Can you work these out from the drawing? Everything is in mm from the part's minimum corner. Round coordinates to 2 decimals unless told otherwise and drop trailing zeros. Loops run counter-clockwise (first coordinate to the right, second up) from the corner with the lowest first, then second, coordinate; pieces in that order, holes last. Notation, with made-up numbers: M 87.25,7 L 118.25,7 A31 cw 118.25,41 Z; hole C -27.5,62 d2. An arc over 180 degrees is marked long. Use a Markdown table: item, result.
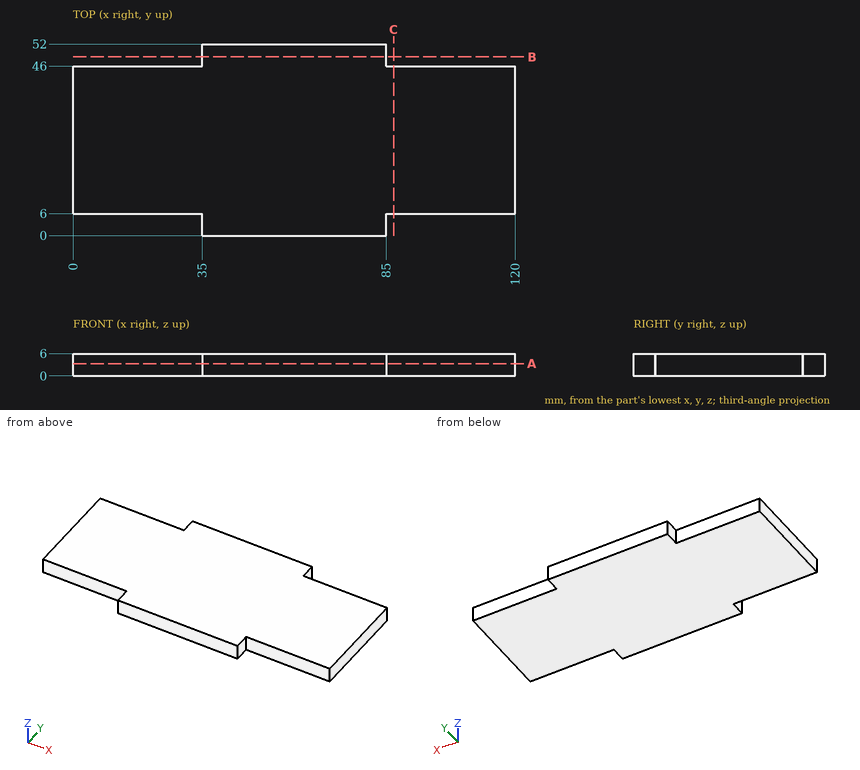
1. I need wall thicknesses on probe 1 along Y at (x, z) = (103, 4.15). Which ranges of the line are inside material? Lowest first, please. Write a range as from..to.
Answer sheet:
| item | result |
|---|---|
| probe 1 | 6..46 |
2. For pin 1 Ø3 at (x, z) = (9, 4.5) entering from -Y; pin 2 Ø3 at (y, z) = (48, 3) entering from -X; pin 3 Ø1 at (x, z) = (103.5, 2.5) entering from +Y, each with a flat end and sliding along its axis, tell me the tip position at first contact or that it passes through.
Answer sheet:
| item | result |
|---|---|
| pin 1 | y = 6 |
| pin 2 | x = 35 |
| pin 3 | y = 46 |
3. Imagine slicing it at B-B, the plane y = 48.5. Write out the boundary of the cut face in (x, z), then the cut area to 3 significant figures.
Answer sheet:
| item | result |
|---|---|
| outline | M 35,0 L 85,0 L 85,6 L 35,6 Z |
| area | 300 mm2 |
4. Imagine slicing it at C-C, the plane x = 87. Write out the boundary of the cut face in (y, z), then the cut area to 3 significant figures.
Answer sheet:
| item | result |
|---|---|
| outline | M 6,0 L 46,0 L 46,6 L 6,6 Z |
| area | 240 mm2 |
5. Imagine slicing it at A-A, the plane z = 3.3. Write out the boundary of the cut face in (x, y).
Answer sheet:
| item | result |
|---|---|
| outline | M 0,6 L 35,6 L 35,0 L 85,0 L 85,6 L 120,6 L 120,46 L 85,46 L 85,52 L 35,52 L 35,46 L 0,46 Z |
